Part model, mm, in its own coordinate system. Face numbers are marked on the shaded views. A direction names the side the tool comes from. Give positions to 0.01 mm unless a question says otherwise; leave off trailing zeros. Write each loop counter-clockwise with the first axis right and the second up, starting at its lowest first coordinate (ties: lowest second). Pieces come first, ordered by that corner, then holes.
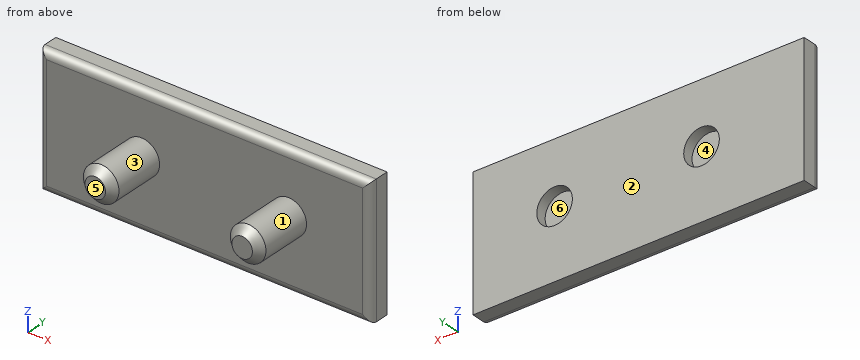
from build123d import *

# Parameters (mm, degrees)
F0_W     = 222.068578
F0_H     = 87.902144
F0_R     = 11.937119
F0_R_2   = 11.938
F1_DEPTH = 7.112
F2_R     = 5.08
F3_DEPTH = 46.736
F4_SIZE  = 5.08


with BuildPart() as f1:
    # F0 (on Front) → F1 (new body, symmetric)
    with BuildSketch(Plane.XZ):
        with Locations((8.572504, -7.892143)):
            Rectangle(F0_W, F0_H)
        with Locations((-33.609644, -5.306785)):
            Circle(F0_R, mode=Mode.SUBTRACT)
        with Locations((64.906068, -5.306785)):
            Circle(F0_R_2, mode=Mode.SUBTRACT)
    extrude(amount=F1_DEPTH, both=True)

    # F2
    f2_edges = [f1.edges().sort_by_distance(p)[0] for p in [
        (8.572504, -7.112, 36.058929),
        (-102.461785, -7.112, -7.892143),
        (8.572504, -7.112, -51.843215),
        (119.606793, -7.112, -7.892143),
    ]]
    fillet(f2_edges, radius=F2_R)

    # F0 (on Front) → F3 (join)
    with BuildSketch(Plane.XZ):
        with Locations((64.906068, -5.306785)):
            Circle(F0_R_2)
        with Locations((-33.609644, -5.306785)):
            Circle(F0_R)
    extrude(amount=F3_DEPTH)

    # F4
    f4_edges = [f1.edges().sort_by_distance(p)[0] for p in [
        (-45.546762, -46.736, -5.306785),
        (52.968068, -46.736, -5.306785),
    ]]
    chamfer(f4_edges, length=F4_SIZE)


solid = f1.part
1) Mould opens along Z. For the marked faces 3, 4, 5 and 6 say: +Z half, -Z half, draft (parallel to the pull), parting line (faces both ways), or undercut.
Check result:
face 3: parting line
face 4: undercut
face 5: draft
face 6: undercut
2) Drill centre lines: L1, parallel to Y at x = 76, z = -11; L2, parallel to X at y = -2.5, z = -25; L3, parallel to X at y = -15.5, z = -11. Where is each one in solid material? Low to high.
Check result:
L1: y = -7.11 to 7.11
L2: x = -102.44 to 119.59
L3: x = -44.1 to -23.12, 54.41 to 75.4
3) 3-axis set-ups, long thin cutter, end or side, ignore diameter. For the marked faces 1 and 2: which of +Z, -Z, +X, -X, +Y, -Y reach the whole face in a straight line?
Check result:
face 1: -Y
face 2: +Z, -Z, +X, -X, +Y
4) Saw through at B-B (y = -16). Write the cut outline in (x, z), and give its area (3 significant figures).
Check result:
outline: circle Ø23.87 at (-33.61, -5.31); circle Ø23.88 at (64.91, -5.31)
area: 895 mm2
5) Saw through at C-C (x = 102). Write the cut outline in (y, z).
Check result:
outline: (-7.11, -46.76) arc R5.08 ccw to (-2.03, -51.84) - (7.11, -51.84) - (7.11, 36.06) - (-2.03, 36.06) arc R5.08 ccw to (-7.11, 30.98) - close
6) Saw through at A-A (z = -36.5). Write the cut outline in (x, y), and give its area (3 significant figures).
Check result:
outline: (-102.46, -2.03) arc R5.08 ccw to (-97.38, -7.11) - (114.53, -7.11) arc R5.08 ccw to (119.61, -2.03) - (119.61, 7.11) - (-102.46, 7.11) - close
area: 3,150 mm2
7) Flat gauge pins, fed straight in: P1, Ø23.5, axis at x = -13, z = 8.5, coming from the -Y side; P2, Ø1, axis at x = 59, z = -0.5, coming from the +Y side; P3, Ø4, axis at x = 66, y = -29, coming from the +Z side. Where does each tip first touch, or does it go through?
Check result:
P1: stops at y = -7.11
P2: stops at y = 0
P3: stops at z = 6.63
